from build123d import *

# Parameters (mm, degrees)
BOSS_EXTRUDE1_DEPTH = 40


with BuildPart() as part:
    # Sketch1 → Boss-Extrude1 (new body)
    with BuildSketch(Plane.XY):
        Polygon((-100, 4.308297624), (-97.5, 14.308297624), (-95, 4.308297624), (-92.5, 14.308297624), (-90, 4.308297624), (-87.5, 14.308297624), (-85, 4.308297624), (-82.5, 14.308297624), (-80, 4.308297624), (-77.5, 14.308297624), (-75, 4.308297624), (-72.5, 14.308297624), (-70, 4.308297624), (-67.5, 14.308297624), (-65, 4.308297624), (-62.5, 14.308297624), (-60, 4.308297624), (-57.5, 14.308297624), (-55, 4.308297624), (-52.5, 14.308297624), (-50, 4.308297624), (-47.5, 14.308297624), (-45, 4.308297624), (-42.5, 14.308297624), (-40, 4.308297624), (-37.5, 14.308297624), (-35, 4.308297624), (-32.5, 14.308297624), (-30, 4.308297624), (-27.5, 14.308297624), (-25, 4.308297624), (-22.5, 14.308297624), (-20, 4.308297624), (-17.5, 14.308297624), (-15, 4.308297624), (-12.5, 14.308297624), (-10, 4.308297624), (-7.5, 14.308297624), (-5, 4.308297624), (-2.5, 14.308297624), (0, 4.308297624), (2.5, 14.308297624), (5, 4.308297624), (7.5, 14.308297624), (10, 4.308297624), (12.5, 14.308297624), (15, 4.308297624), (17.5, 14.308297624), (20, 4.308297624), (22.5, 14.308297624), (25, 4.308297624), (27.5, 14.308297624), (30, 4.308297624), (32.5, 14.308297624), (35, 4.308297624), (37.5, 14.308297624), (40, 4.308297624), (42.5, 14.308297624), (45, 4.308297624), (47.5, 14.308297624), (50, 4.308297624), (52.5, 14.308297624), (55, 4.308297624), (57.5, 14.308297624), (60, 4.308297624), (62.5, 14.308297624), (65, 4.308297624), (67.5, 14.308297624), (70, 4.308297624), (72.5, 14.308297624), (75, 4.308297624), (77.5, 14.308297624), (80, 4.308297624), (82.5, 14.308297624), (85, 4.308297624), (87.5, 14.308297624), (90, 4.308297624), (92.5, 14.308297624), (95, 4.308297624), (97.5, 14.308297624), (100, 4.308297624), (100, -4.308297624), (-100, -4.308297624), align=None)
    extrude(amount=BOSS_EXTRUDE1_DEPTH)


solid = part.part
Can you work these out from the model? Positions are in its coordinate system, mm. Coordinates: 2 decimals unless noted, no trailing zeros. Return JSON: item names as keys, results as strings. Group by question number.
Item 1: If we section it at A-A (y = 8.5): Count the separate pieces of the cut face and the enclosed holes in it, then the cut area to 3 significant figures.
Item 2: I'm going to push flat-ended pins straight in: pin 1 Ø4 at (y, z) = (7.5, 10) entering from +X; pin 2 Ø5 at (y, z) = (7.5, 20) entering from +X. Where does each tip first touch, or does it pass through?
Item 3: We'd pull the mould along X, two halves only. Please class faces 1 (the face through (100, 0, 20)), 2 (the face through (-26.268, 9.378, 19.72)): pulls with the +X half, pulls with the -X half, needs draft (parallel to the pull), parting line crosses it, or undercut.
Return value:
{
 "1": {"separate pieces": "40", "enclosed holes": "0", "area": "4,650 mm^2"},
 "2": {"pin 1": "stops at x = 99.7", "pin 2": "stops at x = 99.83"},
 "3": {"face 1": "pulls with the +X half", "face 2": "undercut"}
}
